Design review of the part shown in the three views and the two pictorial views. Dimensions are in mm from the part's minimum x, y and z. Coordinates: 2 decimals unless noted, no trailing zeros. Loops run counter-clockwise (first coordinate to the right, second up) from the corner with the lowest first, then second, coordinate; pieces in that order, holes last. Notation, with made-up numbers: M 85,-2 L 138,-2 A25 cw 138,16 Z; hole C 82,43 d2. An arc over 180 degrees is marked long. Write item = value, one per line. Start each with the question number.
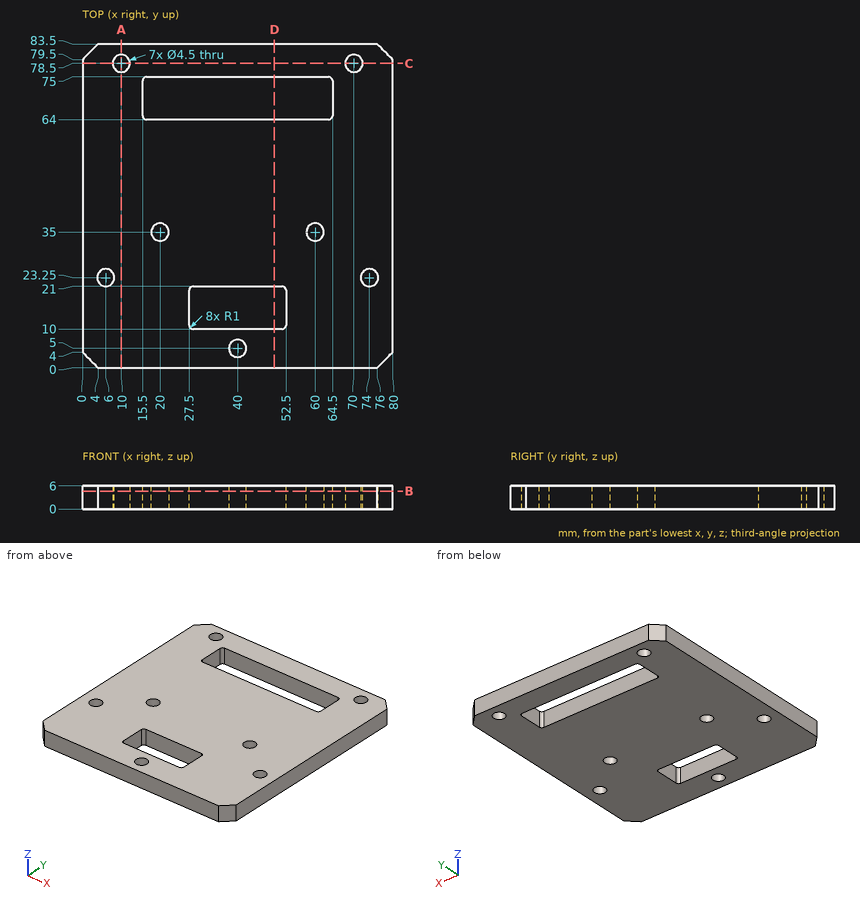
(1) To check wall thickness, follow L1, parallel to Y at x = 40, z = 4.3; L2, parallel to Y at x = 60, z = 1.7; L3, parallel to X at y = 23, z = 2.2. State the ranges of each line that lie inside material, in increasing order.
(2) Take a section at D-D (x = 49.5). State the section outline as (y, z) points, plus the area to 3 significant figures.
(3) Take a section at C-C (y = 78.5). State the section outline as (x, z) points.
(4) Take a section at A-A (x = 10). State the section outline as (y, z) points.
(5) Take a section at B-B (z = 4.65). Give the number of separate pieces and of enclosed holes in the cut face, plus the area to 3 significant figures.
(6) Insertion check: pin 1 (3.5 mm diameter, centred on x = 10, y = 78.5, fed in from -Z). The pin has a flat end and moves straight along its axis. Give the tip position at first contact, or say it passes through.
Results list:
q1.L1 = 0 to 2.75, 7.25 to 10, 21 to 64, 75 to 83.5
q1.L2 = 0 to 32.75, 37.25 to 64, 75 to 83.5
q1.L3 = 0 to 3.76, 8.24 to 71.76, 76.24 to 80
q2.outline = M 0,0 L 10,0 L 10,6 L 0,6 Z; M 21,0 L 64,0 L 64,6 L 21,6 Z; M 75,0 L 83.5,0 L 83.5,6 L 75,6 Z
q2.area = 369 mm^2
q3.outline = M 0,0 L 7.75,0 L 7.75,6 L 0,6 Z; M 12.25,0 L 67.75,0 L 67.75,6 L 12.25,6 Z; M 72.25,0 L 80,0 L 80,6 L 72.25,6 Z
q4.outline = M 0,0 L 76.25,0 L 76.25,6 L 0,6 Z; M 80.75,0 L 83.5,0 L 83.5,6 L 80.75,6 Z
q5.separate_pieces = 1
q5.enclosed_holes = 9
q5.area = 5,720 mm^2
q6.pin_1 = through
